Autodesk Inventor part; units mm, degrees
ref_plane "Plano de trabajo1" through (0, 23, 5) normal (0, 0, 1) x (1, 0, 0)
ref_plane "YZ Plane" through (0, 0, 0) normal (1, 0, 0) x (0, 1, 0)
ref_plane "XZ Plane" through (0, 0, 0) normal (0, 1, 0) x (-1, 0, 0)
sketch "Boceto1" plane through (0, 0, 0) normal (0, 1, 0) x (-1, 0, 0)
  circle A0 centre (0, 0) radius 5
  dimension "d0" = 10
extrude "Extrusión1" add sketch "Boceto1" along normal blind 21
thread "Rosca1"
sketch "Boceto2" plane through (0, 21, 0) normal (0, 1, 0) x (1, 0, 0)
  circle A0 centre (0, 0) radius 6
  dimension "d5" = 12
extrude "Extrusión2" add sketch "Boceto2" along normal blind 2
sketch "Boceto3" plane through (0, 23, 0) normal (0, 1, 0) x (1, 0, 0)
  circle A0 centre (0, 0) radius 5
  dimension "d8" = 10
extrude "Extrusión3" add sketch "Boceto3" along normal blind 10
ref_plane "Plano de trabajo1" through (0, 23, 5) normal (0, 0, 1) x (1, 0, 0)
sketch "Boceto4" plane through (0, 23, 5) normal (0, 0, 1) x (1, 0, 0)
  line L0 (5, 10) -> (-5, 10)
  line L1 (-5, 10) -> (5.0514, 0) construction
  line L2 (6, 0) -> (-6, 0)
  line L3 (5, 0) -> (5, 10)
  line L4 (5, 10) -> (-4.9489, 0) construction
  circle A0 centre (0.0256, 5) radius 2.5
  point P0 (0, -23)
  dimension "d11" = 5
extrude "Extrusión4" cut sketch "Boceto4" against normal through all
Source: CAD feature listing. Evaluate the final solid. Frame: model axes, mm. A direction names the side the tool comes from. Coordinates: 2 decimals unless noted, no trailing zeros. Loops run counter-clockwise (first coordinate to the right, second up) from the corner with the lowest first, then second, coordinate; pieces in that order, holes last. Notation, with made-up numbers: (47, 52.5) -> (68, 52.5) arc R17 ccw to (68, 79.5) -> close; hole circle Ø5 at (50.5, 27.25). An arc over 180 degrees is marked (long way). One line per item, written item: value. Start each with the question number.
Q1. Section query A-A, the plane z = 0. Return the cut outline in (x, y).
Q2. Section query D-D, the plane z = 2.25. Return the cut outline in (x, y), and give its area (3 significant figures).
Q3. Line query: line 1 along X through (y, z) = (28, 0.25); line 2 along X through (y, z) = (12, -0.25); line 3 along X through (y, z) = (27, -3.5). Output: solid intervals per line, ascending.
Q4. Mould query, pull axis X, two halves, no side actions, for faces 1 (the face through (2.41, 28.75, 0.07)), 2 (the face through (-6, 22, 0)), 3 (the face through (0, 33, 0)). Classes: pulls with the +X half, pulls with the -X half, needs draft (parallel to the pull), parting line crosses it, or undercut.
Q5. Section query C-C, the plane y = 3. Return the cut outline in (x, z), and give its area (3 significant figures).
Q6. Set-up query: faces 4 (the face through (1.08, 10.35, 4.88)), 5 (the face through (-4, 23, -4)), 6 (the face through (0, 0, 0)). Return all of +Z, -Z, +X, -X, +Y, -Y with unobstructed straight access to the full face (end or side cutting, diameter ignored); none if empty.
Q7. Section query B-B, the plane x = 0. Return the cut outline in (y, z), and give its area (3 significant figures).
Q8. Contact query for flat-ended pins moving along their axis: P1, Ø4, axis at y = 8, z = 4, coming from the -X side; P2, Ø6.5, axis at x = 0.03, y = 28, coming from the -Z side; P3, Ø6, axis at y = 8.5, z = -1, coming from the -X side. Output: stop coordinate, or through.
Results:
1. outline: (-6, 21) -> (-5, 21) -> (-5, 0) -> (5, 0) -> (5, 21) -> (6, 21) -> (6, 23) -> (5, 23) -> (5, 33) -> (-5, 33) -> (-5, 23) -> (-6, 23) -> close; hole circle Ø5 at (0.03, 28)
2. outline: (-5.56, 21) -> (-4.47, 21) -> (-4.47, 0) -> (4.47, 0) -> (4.47, 21) -> (5.56, 21) -> (5.56, 23) -> (4.47, 23) -> (4.47, 33) -> (-4.47, 33) -> (-4.47, 23) -> (-5.56, 23) -> close; hole circle Ø5 at (0.03, 28)
2. area: 279 mm^2
3. line 1: -4.99 to -2.47, 2.53 to 4.99
3. line 2: -4.99 to 4.99
3. line 3: -3.57 to -2.27, 2.32 to 3.57
4. face 1: undercut
4. face 2: parting line crosses it
4. face 3: needs draft
5. outline: circle Ø10 at (0, 0)
5. area: 78.5 mm^2
6. face 4: -Y
6. face 5: +Y
6. face 6: +Z, -Z, +X, -X, -Y
7. outline: (0, -5) -> (21, -5) -> (21, -6) -> (23, -6) -> (23, -5) -> (25.5, -5) -> (25.5, 5) -> (23, 5) -> (23, 6) -> (21, 6) -> (21, 5) -> (0, 5) -> close; (30.5, -5) -> (33, -5) -> (33, 5) -> (30.5, 5) -> close
7. area: 284 mm^2
8. P1: x = -4.58
8. P2: z = -5
8. P3: x = -5
